Check sheet for the modelled part. Datum: model origin and axes. Units: mm. Face numbers are marked on the shaded views. Give positions to 0.01 mm unless a question says otherwise; leave off trailing zeros. Loops run counter-clockwise (first coordinate to the right, second up) from the corner with the lowest first, then second, coordinate; pieces in that order, holes last.
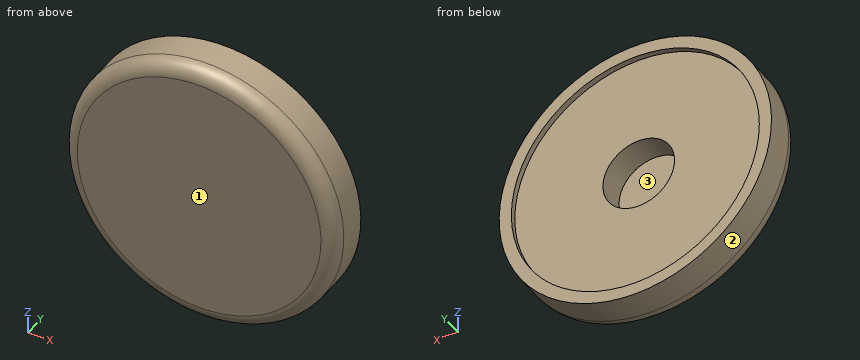
```python
from build123d import *

# Parameters (mm, degrees)
SKETCH2_R           = 24.13
BOSS_EXTRUDE1_DEPTH = 7.62
SKETCH3_R           = 21.971
CUT_EXTRUDE1_DEPTH  = 1.016
SKETCH4_R           = 6.35
CUT_EXTRUDE2_DEPTH  = 4.826
FILLET1_R           = 2.54


with BuildPart() as part:
    # Sketch2 → Boss-Extrude1 (new body)
    with BuildSketch(Plane(origin=(0, 0, 0), x_dir=(1, 0, 0), z_dir=(0, 1, 0))):
        with Locations(Location((0, 0, 0), (0, 0, 90))):
            Circle(SKETCH2_R)
    extrude(amount=BOSS_EXTRUDE1_DEPTH)

    # Sketch3 → Cut-Extrude1 (cut)
    with BuildSketch(Plane(origin=(0, 7.62, 0), x_dir=(1, 0, 0), z_dir=(0, 1, 0))):
        with Locations(Location((0, 0, 0), (0, 0, 270))):
            Circle(SKETCH3_R)
    extrude(amount=-CUT_EXTRUDE1_DEPTH, mode=Mode.SUBTRACT)

    # Sketch4 → Cut-Extrude2 (cut)
    with BuildSketch(Plane(origin=(0, 6.604, 0), x_dir=(1, 0, 0), z_dir=(0, 1, 0))):
        with Locations(Location((0, 0, 0), (0, 0, 270))):
            Circle(SKETCH4_R)
    extrude(amount=-CUT_EXTRUDE2_DEPTH, mode=Mode.SUBTRACT)

    # Fillet1
    fillet1_edges = [part.edges().sort_by_distance(p)[0] for p in [
        (0, 0, 24.13),
    ]]
    fillet(fillet1_edges, radius=FILLET1_R)


solid = part.part
```
(1) Section check A-A on x = 0. Record the boundary of the cut face in (y, z).
(2) Section check C-C on y = 4.75. Record the boundary of the cut face in (x, z), plus the area to 3 significant figures.
(3) Material ranges on line 1 (X direction, y = 7, z = 0); line 2 (X direction, y = 5.5, z = 0); line 3 (Y direction, x = -1.5, z = 14.5), recorded low to high.
(4) Gauge pin test, flat ends, axial feed: pin 1 Ø1 at (x, z) = (19, 3.5) entering from +Y; pin 2 Ø4 at (x, z) = (0.5, 2) entering from +Y; pin 3 Ø1.5 at (y, z) = (6.5, -19) entering from -X. Record the tip position at first contact, or that the pin passes through.
(5) Section check B-B on z = 0. Record the boundary of the cut face in (x, y), plus the area to 3 significant figures.
(6) Release check for a two-part mould opening along Z. For the marked faces 1, 2 and 3 record: pulls with the +Z half, pulls with the -Z half, needs draft (parallel to the pull), parting line crosses it, or undercut.
Computed values:
1. outline: (0, -21.59) arc R2.54 ccw to (2.54, -24.13) - (7.62, -24.13) - (7.62, -21.97) - (6.6, -21.97) - (6.6, -6.35) - (1.78, -6.35) - (1.78, 6.35) - (6.6, 6.35) - (6.6, 21.97) - (7.62, 21.97) - (7.62, 24.13) - (2.54, 24.13) arc R2.54 ccw to (0, 21.59) - close
2. outline: circle Ø48.26 at (0, 0); hole circle Ø12.7 at (0, 0)
2. area: 1,700 mm2
3. line 1: x = -24.13 to -21.97, 21.97 to 24.13
3. line 2: x = -24.13 to -6.35, 6.35 to 24.13
3. line 3: y = 0 to 6.6
4. pin 1: stops at y = 6.6
4. pin 2: stops at y = 1.78
4. pin 3: stops at x = -15.79
5. outline: (-24.13, 2.54) arc R2.54 ccw to (-21.59, 0) - (21.59, 0) arc R2.54 ccw to (24.13, 2.54) - (24.13, 7.62) - (21.97, 7.62) - (21.97, 6.6) - (6.35, 6.6) - (6.35, 1.78) - (-6.35, 1.78) - (-6.35, 6.6) - (-21.97, 6.6) - (-21.97, 7.62) - (-24.13, 7.62) - close
5. area: 259 mm2
6. face 1: needs draft
6. face 2: parting line crosses it
6. face 3: undercut
